Part model, mm, in its own coordinate system. A direction names the side the tool comes from. Give positions to 0.01 mm unless a question says otherwise; leave off trailing zeros. Write each loop counter-clockwise with the first axis right and the second up, starting at its lowest first coordinate (ties: lowest second). Pieces come first, ordered by that corner, then holes.
from build123d import *

# Parameters (mm, degrees)
SKETCH1_R                 = 19
BOSS_EXTRUDE1_DEPTH       = 4
M4_CLEARANCE_HOLE1_D      = 4.5
BOSS_EXTRUDE2_DEPTH       = 17
CHAMFER1_SIZE             = 0.5
M3X0_5_TAPPED_HOLE1_D     = 2.5
M3X0_5_TAPPED_HOLE1_DEPTH = 7.5
M3X0_5_TAPPED_HOLE1_TIP   = 0.751075774


with BuildPart() as part:
    # Sketch1 → Boss-Extrude1 (new body)
    with BuildSketch(Plane.XY):
        Circle(SKETCH1_R)
    extrude(amount=BOSS_EXTRUDE1_DEPTH)

    # M4 Clearance Hole1 (through all)
    with Locations(Plane.XY.offset(4)):
        with Locations((10.606601718, 10.606601718), (-10.606601718, -10.606601718), (-10.606601718, 10.606601718), (10.606601718, -10.606601718)):
            Hole(M4_CLEARANCE_HOLE1_D / 2)

    # Sketch4 → Boss-Extrude2 (add)
    with BuildSketch(Plane.XY.offset(4)):
        with BuildLine():
            Line((-3, -4), (3, -4))
            ThreePointArc((3, -4), (5.121320344, -3.121320344), (6, -1))
            Line((6, -1), (6, 1))
            ThreePointArc((6, 1), (5.121320344, 3.121320344), (3, 4))
            Line((3, 4), (-3, 4))
            ThreePointArc((-3, 4), (-5.121320344, 3.121320344), (-6, 1))
            Line((-6, 1), (-6, -1))
            ThreePointArc((-6, -1), (-5.121320344, -3.121320344), (-3, -4))
        make_face()
    extrude(amount=BOSS_EXTRUDE2_DEPTH)

    # Chamfer1
    chamfer1_edges = [part.edges().sort_by_distance(p)[0] for p in [
        (5.121320344, 3.121320344, 21),
        (0, 4, 21),
        (-5.121320344, 3.121320344, 21),
        (-6, 0, 21),
        (-5.121320344, -3.121320344, 21),
        (0, -4, 21),
        (5.121320344, -3.121320344, 21),
        (6, 0, 21),
    ]]
    chamfer(chamfer1_edges, length=CHAMFER1_SIZE)

    # M3x0.5 Tapped Hole1
    with Locations(Plane.XY.offset(21)):
        with Locations((-2.5, 0), (2.5, 0)):
            Hole(M3X0_5_TAPPED_HOLE1_D / 2, depth=M3X0_5_TAPPED_HOLE1_DEPTH)
            with Locations((0, 0, -(M3X0_5_TAPPED_HOLE1_DEPTH + M3X0_5_TAPPED_HOLE1_TIP / 2))):  # 118° drill point
                Cone(0, M3X0_5_TAPPED_HOLE1_D / 2, M3X0_5_TAPPED_HOLE1_TIP, mode=Mode.SUBTRACT)


solid = part.part
1) Saw through at B-B (x = 0). Write the cut outline in (y, z).
Check result:
outline: (-19, 0) - (19, 0) - (19, 4) - (4, 4) - (4, 20.5) - (3.5, 21) - (-3.5, 21) - (-4, 20.5) - (-4, 4) - (-19, 4) - close
2) 3-axis set-ups, long thin cutter, end or side, ignore diameter. For faces 4 (the flat face through (-6, 0, 12)), 5 (the cylindrical face through (5.14, 3.1, 12.13)), 6 (the cylindrical face through (5.1, -3.14, 12.13)): which of +Z, -Z, +X, -X, +Y, -Y reach the whole face in a straight line?
Check result:
face 4: +Z, -X, +Y, -Y
face 5: +Z, +X, +Y
face 6: +Z, +X, -Y
3) Mould opens along X. For faces 1 (the conical face through (2.28, 0.01, 12.88)), 2 (the flat face through (6, 0, 12)), 3 (the flat face through (0, 4, 12)) say: +X half, -X half, draft (parallel to the pull), parting line (faces both ways), or undercut.
Check result:
face 1: undercut
face 2: +X half
face 3: draft
4) Drill centre lines: L1, parallel to X at y = 0, z = 17.25; L2, parallel to Y at x = -2.5, z = 15.5; L3, parallel to Z at x = 4, y = -9. Where is each one in solid material? Low to high.
Check result:
L1: x = -6 to -3.75, -1.25 to 1.25, 3.75 to 6
L2: y = -4 to -1.25, 1.25 to 4
L3: z = 0 to 4
5) Flat gauge pins, fed straight in: P1, Ø1, axis at y = 0, z = 13, coming from the +X side; P2, Ø1.5, axis at x = -2, z = 13.5, coming from the +Y side; P3, Ø0.6, axis at y = 0.5, z = 11.5, coming from the -X side. Where does each tip first touch, or does it go through?
Check result:
P1: stops at x = 6
P2: stops at y = 4
P3: stops at x = -6
6) Saw through at A-A (z = 16). Write the cut outline in (x, y), and give its area (3 significant figures).
Check result:
outline: (-6, -1) arc R3 ccw to (-3, -4) - (3, -4) arc R3 ccw to (6, -1) - (6, 1) arc R3 ccw to (3, 4) - (-3, 4) arc R3 ccw to (-6, 1) - close; hole circle Ø2.5 at (-2.5, 0); hole circle Ø2.5 at (2.5, 0)
area: 78.5 mm2
7) Saw through at C-C (z = 8.25). Write the cut outline in (x, y), and give its area (3 significant figures).
Check result:
outline: (-6, -1) arc R3 ccw to (-3, -4) - (3, -4) arc R3 ccw to (6, -1) - (6, 1) arc R3 ccw to (3, 4) - (-3, 4) arc R3 ccw to (-6, 1) - close
area: 88.3 mm2
8) Saw through at D-D (z = 2.75). Write the cut outline in (x, y).
Check result:
outline: circle Ø38 at (0, 0); hole circle Ø4.5 at (-10.61, -10.61); hole circle Ø4.5 at (-10.61, 10.61); hole circle Ø4.5 at (10.61, -10.61); hole circle Ø4.5 at (10.61, 10.61)
